Verification items for the finished model (mm, model axes). A direction names the side the tool comes from. Round coordinates to 2 decimals unless told otherwise and drop trailing zeros. Write each loop counter-clockwise with the first axis right and the second up, starting at its lowest first coordinate (ties: lowest second). Pieces come first, ordered by that corner, then holes. Notation, with made-up numbers: (88, -5.75) - (133, -5.75) arc R17 cw to (133, 5.25) - close; hole circle Ø4 at (74.25, 53.5). An arc over 180 degrees is marked (long way). Answer as a JSON object with one key per item and string values.
Autodesk Inventor part; units mm, degrees
ref_plane "工作平面1" through (0, 0, 0) normal (0, 0, 1) x (1, 0, 0)
ref_plane "工作平面2" through (28.2, -16.65, -54) normal (1, 0, 0) x (0, 1, 0)
ref_plane "工作平面3" through (48, 0, 0) normal (1, 0, 0) x (0, 1, 0)
sketch "草圖1" plane through (0, 0, 0) normal (0, 0, 1) x (1, 0, 0)
  circle A0 centre (0, 0) radius 60
  circle A1 centre (0, 0) radius 48
  dimension "d0" = 120
  dimension "d1" = 96
extrude "擠出1" add sketch "草圖1" along normal blind 27.1 and the other way blind 60
sketch "草圖2" plane through (0, 0, 27.1) normal (0, 0, 1) x (1, 0, 0)
  circle A0 centre (0, 0) radius 54 construction
  circle A1 centre (0, 54) radius 2.5
  circle A2 centre (-54, 0) radius 2.5
  circle A3 centre (0, -54) radius 2.5
  circle A4 centre (54, 0) radius 2.5
  dimension "d6" = 108
  dimension "d7" = 5
  dimension "d10" = 360
extrude "擠出2" cut sketch "草圖2" against normal blind 20
ref_plane "工作平面1" through (0, 0, 0) normal (0, 0, 1) x (1, 0, 0)
sketch "草圖3" plane through (0, 0, 0) normal (0, 0, 1) x (1, 0, 0)
  circle A0 centre (-23.57, 23.57) radius 2.3
  circle A1 centre (23.57, 23.57) radius 2.3
  circle A2 centre (23.57, -23.57) radius 2.3
  circle A3 centre (-23.57, -23.57) radius 2.3
  circle A4 centre (-23.57, 23.57) radius 2.7
  circle A5 centre (23.57, 23.57) radius 2.7
  circle A6 centre (23.57, -23.57) radius 2.7
  circle A7 centre (-23.57, -23.57) radius 2.7
  circle A8 centre (0, 0) radius 22.5
  line L0 (-21.9436, 4.973) -> (-41.3486, 24.3781)
  circle A9 centre (0, 0) radius 48
  line L1 (-24.3781, 41.3486) -> (-4.973, 21.9436)
  line L2 (-23.57, 23.57) -> (0, 0) construction
  circle A10 centre (0, 0) radius 40.5
  line L3 (-41.3486, -24.3781) -> (-21.9436, -4.973)
  line L4 (-4.973, -21.9436) -> (-24.3781, -41.3486)
  line L5 (24.3781, -41.3486) -> (4.973, -21.9436)
  line L6 (21.9436, -4.973) -> (41.3486, -24.3781)
  line L7 (41.3486, 24.3781) -> (21.9436, 4.973)
  line L8 (4.973, 21.9436) -> (24.3781, 41.3486)
  point P0 (-18.8666, 35.8372)
  point P1 (-35.8372, 18.8666)
  point P2 (-35.8372, -18.8666)
  point P3 (-24.3781, -41.3486)
  point P4 (-18.8666, -35.8372)
  point P5 (18.8666, -35.8372)
  point P6 (24.3781, -41.3486)
  point P7 (41.3486, -24.3781)
  point P8 (35.8372, -18.8666)
  point P9 (35.8372, 18.8666)
  point P10 (41.3486, 24.3781)
  point P11 (24.3781, 41.3486)
  point P12 (18.8666, 35.8372)
  dimension "d14" = 5.4
  dimension "d15" = 5.4
  dimension "d16" = 5.4
  dimension "d17" = 5.4
  dimension "d18" = 45
  dimension "d19" = 24
  dimension "d20" = 12
  dimension "d21" = 18
  dimension "d24" = 360
extrude "擠出3" add sketch "草圖3" along normal blind 5 contours A8 L7 A10 L6 | A8 L8 A10 L7 | L6 A10 L5 A8 | A8 L1 A10 L8 | A10 L8 A9 L7 | L5 A10 L4 A8 | L6 A9 L5 A10 | A8 L0 A10 L1 | L4 A10 L3 A8 | A8 L3 A10 L0 | A10 L0 A9 L1 | L4 A9 L3 A10
sketch "草圖4" plane through (0, 0, -60) normal (0, 0, -1) x (-1, 0, 0)
  circle A0 centre (0, 0) radius 54 construction
  circle A1 centre (0, -54) radius 2.5
  circle A2 centre (46.7654, -27) radius 2.5
  circle A3 centre (46.7654, 27) radius 2.5
  circle A4 centre (0, 54) radius 2.5
  circle A5 centre (-46.7654, 27) radius 2.5
  circle A6 centre (-46.7654, -27) radius 2.5
  dimension "d29" = 108
  dimension "d32" = 360
  dimension "d62" = 5
extrude "擠出4" cut sketch "草圖4" against normal blind 20
ref_plane "工作平面2" through (28.2, -16.65, -54) normal (1, 0, 0) x (0, 1, 0)
sketch "草圖5" plane through (28.2, -16.65, -54) normal (1, 0, 0) x (0, 1, 0)
  circle A0 centre (16.65, 14) radius 5
  line L0 (-43.35, -6) -> (76.65, -6)
  point P0 (16.65, 54)
  dimension "d36" = 10
  dimension "d37" = 20
extrude "擠出5" cut sketch "草圖5" along normal through all
ref_plane "工作平面3" through (48, 0, 0) normal (1, 0, 0) x (0, 1, 0)
sketch "草圖7" plane through (48, 0, 0) normal (1, 0, 0) x (0, 1, 0)
  line L0 (9, 15.1) -> (-9, 15.1)
  line L1 (-9, 15.1) -> (-9, 8.85)
  line L2 (-9, 8.85) -> (9, 8.85)
  line L3 (9, 8.85) -> (9, 15.1)
  line L4 (-48, 27.1) -> (48, 27.1)
  point P0 (0, 0)
  dimension "d45" = 18
  dimension "d46" = 9
  dimension "d47" = 6.25
  dimension "d48" = 12
extrude "擠出6" add sketch "草圖7" against normal blind 0.85
sketch "草圖8" plane through (47.15, 0, 0) normal (-1, 0, 0) x (0, 0, 1)
  line L0 (15.1, -8.9932) -> (8.85, -8.9932)
  line L1 (15.1, -8.9932) -> (15.1, 8.9932)
  line L2 (8.85, 8.9932) -> (15.1, 8.9932)
  line L3 (8.85, 8.9932) -> (8.85, -8.9932)
  line L4 (15.1, 0) -> (8.85, 0)
  circle A0 centre (11.975, 5.75) radius 1.6
  circle A1 centre (11.975, -5.75) radius 1.6
  point P0 (0, 0)
  point P1 (11.975, 8.9932)
  dimension "d52" = 3.2
  dimension "d53" = 5.75
extrude "擠出7" cut sketch "草圖8" against normal through all contours A0 | A1
sketch "草圖9" plane through (0, 0, 5) normal (0, 0, 1) x (1, 0, 0)
  line L0 (-24.3781, -41.3486) -> (-18.8666, -35.8372)
  arc A0 (-18.8666, -35.8372) -> (18.8666, -35.8372) centre (0, 0) ccw
  line L1 (18.8666, -35.8372) -> (24.3781, -41.3486)
  line L2 (41.3486, -24.3781) -> (35.8372, -18.8666)
  arc A1 (35.8372, -18.8666) -> (35.8372, 18.8666) centre (0, 0) ccw
  line L3 (35.8372, 18.8666) -> (41.3486, 24.3781)
  line L4 (24.3781, 41.3486) -> (18.8666, 35.8372)
  arc A2 (18.8666, 35.8372) -> (-18.8666, 35.8372) centre (0, 0) ccw
  line L5 (-18.8666, 35.8372) -> (-24.3781, 41.3486)
  line L6 (-41.3486, 24.3781) -> (-35.8372, 18.8666)
  arc A3 (-35.8372, 18.8666) -> (-35.8372, -18.8666) centre (0, 0) ccw
  line L7 (-35.8372, -18.8666) -> (-41.3486, -24.3781)
  circle A4 centre (23.57, -23.57) radius 2.7
  circle A5 centre (23.57, 23.57) radius 2.7
  circle A6 centre (-23.57, 23.57) radius 2.7
  circle A7 centre (-23.57, -23.57) radius 2.7
  circle A8 centre (0, 0) radius 22.5
  line L8 (18.8666, -35.8372) -> (-18.8666, -35.8372)
  line L9 (35.8372, 18.8666) -> (35.8372, -18.8666)
  line L10 (-18.8666, 35.8372) -> (18.8666, 35.8372)
  line L11 (-35.8372, -18.8666) -> (-35.8372, 18.8666)
  arc A9 (-24.3781, 41.3486) -> (-41.3486, 24.3781) centre (0, 0) ccw
  arc A10 (-41.3486, -24.3781) -> (-24.3781, -41.3486) centre (0, 0) ccw
  arc A11 (24.3781, -41.3486) -> (41.3486, -24.3781) centre (0, 0) ccw
  arc A12 (41.3486, 24.3781) -> (24.3781, 41.3486) centre (0, 0) ccw
  point P0 (35.8372, 18.8666)
  point P1 (-18.8666, 35.8372)
  point P2 (-35.8372, -18.8666)
  dimension "d58" = 360
extrude "擠出8" cut sketch "草圖9" against normal up to surface (5 mm away) contours L8 A0 | A3 L11 | L9 A1 | A2 L10
thread "螺紋1"
thread "螺紋2"
thread "螺紋3"
thread "螺紋4"
thread "螺紋5"
thread "螺紋6"
thread "螺紋7"
thread "螺紋8"
thread "螺紋9"
thread "螺紋10"
equation "\"d20\" = 0.5 * d19"
properties part number "j1 57 mount"
Q1. Section check D-D, the plane y = 54. Record the cut outline in (x, z).
Geometry check:
{"outline": "(-26.15, -60) - (-2.5, -60) - (-2.5, -40) - (2.5, -40) - (2.5, -60) - (26.15, -60) - (26.15, 27.1) - (2.5, 27.1) - (2.5, 7.1) - (-2.5, 7.1) - (-2.5, 27.1) - (-26.15, 27.1) - close"}
Q2. Section check B-B, the plane x = 16. Record the cut outline in (y, z), then the cut area to 3 significant figures.
Geometry check:
{"outline": "(-57.83, -60) - (-45.25, -60) - (-45.25, 27.1) - (-57.83, 27.1) - close; (-35.84, 0) - (-15.82, 0) - (-15.82, 5) - (-35.84, 5) - close; (15.82, 0) - (35.84, 0) - (35.84, 5) - (15.82, 5) - close; (45.25, -60) - (57.83, -60) - (57.83, 27.1) - (45.25, 27.1) - close", "area": "2,390 mm2"}
Q3. Section check A-A, the plane z = -54. Record the cut outline in (x, y), then the cut area to 3 significant figures.
Geometry check:
{"outline": "circle Ø120 at (0, 0); hole circle Ø5 at (-46.77, -27); hole circle Ø5 at (-46.77, 27); hole circle Ø96 at (0, 0); hole circle Ø5 at (0, -54); hole circle Ø5 at (0, 54); hole circle Ø5 at (46.77, -27); hole circle Ø5 at (46.77, 27)", "area": "3,950 mm2"}
Q4. Set-up check for faces 1 (the flat face through (-47, 27, -40)), 2 (the flat face through (-38.55, 21.58, 2.46)), 3 (the cylindrical face through (53.414, -6.724, 10.705)), 4 (the cylindrical face through (-0.54, -56.44, 17.24)): record each of +Z, -Z, +X, -X, +Y, -Y from which the full face is reachable in a straight line by a thin tool's end or side.
Geometry check:
{"face 1": "-Z", "face 2": "+Z, -Z", "face 3": "+X", "face 4": "+Z"}
Q5. Material ranges on line 1 along Y through (x, z) = (-23.57, 2.5); line 2 along Y through (x, z) = (0, -3); line 3 along Y through (x, z) = (-23, 1), recorded low to high. Write a range as [from, to].
Geometry check:
{"line 1": "y = [-55.18, -41.81], [-40.54, -26.27], [-20.87, 20.87], [26.27, 40.54], [41.81, 55.18]", "line 2": "y = [-60, -48], [48, 60]", "line 3": "y = [-55.42, -42.13], [-39.97, -26.21], [-20.93, 20.93], [26.21, 39.97], [42.13, 55.42]"}
Q6. Gauge pin test, flat ends, axial feed: P1, Ø4, axis at y = -5.75, z = 11.975, coming from the +X side; P2, Ø6, axis at x = -12.5, y = 25.5, coming from the +Z side; P3, Ø1.5, axis at y = -19.5, z = -3.5, coming from the +X side. Record the tip position at first contact, or that the pin passes through.
Geometry check:
{"P1": "stops at x = 59.88", "P2": "stops at z = 5", "P3": "stops at x = 57"}
Q7. Section check C-C, the plane x = 38.5. Record the cut outline in (y, z), then the cut area to 3 significant figures.
Geometry check:
{"outline": "(-46.02, -60) - (-28.67, -60) - (-28.67, 0) - (-21.53, 0) - (-21.53, 5) - (-28.67, 5) - (-28.67, 27.1) - (-46.02, 27.1) - close; (21.53, 0) - (28.67, 0) - (28.67, -60) - (46.02, -60) - (46.02, 27.1) - (28.67, 27.1) - (28.67, 5) - (21.53, 5) - close", "area": "3,090 mm2"}
